The model under review builds one solid part; all positions refer to its coordinate system, in mm. Face numbers are marked on the shaded views. A direction names the side the tool comes from. Round coordinates to 2 decimals unless told otherwise and drop trailing zeros. Write each loop counter-clockwise with the first axis right and the second up, starting at its lowest first coordinate (ties: lowest second). Pieces come first, ordered by that corner, then holes.
Item 1: Add section C-C (x = -16). Give the boundary of the cut face in (y, z), plus the area to 3 significant figures.
Item 2: Add section A-A (z = 13). Give the boundary of the cut face in (x, y), plus the area to 3 significant figures.
Item 3: Add section B-B (y = 8.75). Give the boundary of the cut face in (x, z).
Item 4: Add section D-D (z = 33). Give the boundary of the cut face in (x, y).
Item 5: Machinability: for the marked faces 1, 2 and 3, which of the approach directions +Z, -Z, +X, -X, +Y, -Y give a long, thin tool a straight path to every point of the face, cutting with its end or side? Answer none if there is none.
Item 6: Clearance check with flat-ended pins moving along their axes: pin 1 Ø11.5 at (x, z) = (-57.5, 15.5) entering from -Y; pin 2 Ø5 at (y, z) = (1.5, 42.5) entering from -X; pin 3 Ø9 at (x, y) = (-95, 9) entering from +Z; pin 4 Ø5 at (y, z) = (1.5, 22) entering from -X. State where each tip first meets the part, or that it passes through.
Item 7: To check wall thickness, follow L1, parallel to X at y = 14.5, z = 41; L2, parallel to Z at x = -39, y = 7.5; L3, parallel to X at y = 9, z = 25. State the ranges of each line that lie inside material, in increasing order.
```python
from build123d import *

# Parameters (mm, degrees)
EXTRUDE_1_DEPTH     = 60
SKETCH_2_W          = 5
SKETCH_2_H          = 8
EXTRUDE_2_DEPTH     = 175
CHAMFER_1_SIZE      = 20
CUT_EXTRUDE_1_DEPTH = 33.8
CHAMFER_2_SIZE      = 2


with BuildPart() as part:
    # 草图1 → 凸台-拉伸1 (new body)
    with BuildSketch(Plane.XY):
        Polygon((5.6, 10.6), (3.2, 10.6), (3.2, 15.2), (0, 15.2), (0, 0), (3.2, 0), (3.2, 4.6), (5.6, 4.6), (5.6, -2.4), (-2.4, -2.4), (-2.4, 17.6), (5.6, 17.6), align=None)
    extrude(amount=EXTRUDE_1_DEPTH)

    # 草图2 → 凸台-拉伸2 (add)
    with BuildSketch(Plane.ZY.offset(2.4)):
        with Locations((2.5, 7.6)):
            Rectangle(SKETCH_2_W, SKETCH_2_H)
    extrude(amount=EXTRUDE_2_DEPTH)

    # 倒角1
    chamfer_1_edges = [part.edges().sort_by_distance(p)[0] for p in [
        (-2.4, 7.6, 5),
    ]]
    chamfer(chamfer_1_edges, length=CHAMFER_1_SIZE)

    # 草图3 → 切除-拉伸1 (cut)
    with BuildSketch(Plane(origin=(0, 11.6, 0), x_dir=(1, 0, 0), z_dir=(0, 1, 0))):
        Polygon((-177.4, -2.5), (-157.4, -5), (-177.4, -5), align=None)
    extrude(amount=-CUT_EXTRUDE_1_DEPTH, mode=Mode.SUBTRACT)

    # 倒角2
    chamfer_2_edges = [part.edges().sort_by_distance(p)[0] for p in [
        (-2.4, 3.6, 12.5),
        (-2.4, 11.6, 12.5),
    ]]
    chamfer(chamfer_2_edges, length=CHAMFER_2_SIZE)


solid = part.part
```
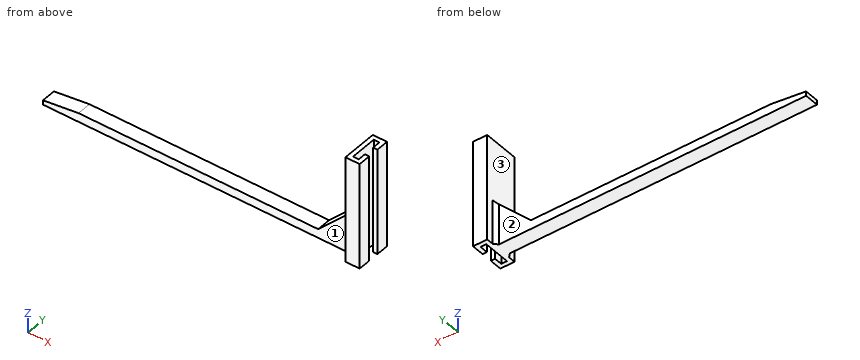
Numbers:
1. outline: (3.6, 0) - (11.6, 0) - (11.6, 11.4) - (3.6, 11.4) - close
1. area: 91.2 mm2
2. outline: (-14.4, 3.6) - (-4.4, 3.6) - (-2.4, 1.6) - (-2.4, -2.4) - (5.6, -2.4) - (5.6, 4.6) - (3.2, 4.6) - (3.2, 0) - (0, 0) - (0, 15.2) - (3.2, 15.2) - (3.2, 10.6) - (5.6, 10.6) - (5.6, 17.6) - (-2.4, 17.6) - (-2.4, 13.6) - (-4.4, 11.6) - (-14.4, 11.6) - close
2. area: 197 mm2
3. outline: (-177.4, 0) - (0, 0) - (0, 60) - (-2.4, 60) - (-2.4, 25) - (-22.4, 5) - (-157.4, 5) - (-177.4, 2.5) - close
4. outline: (-2.4, -2.4) - (5.6, -2.4) - (5.6, 4.6) - (3.2, 4.6) - (3.2, 0) - (0, 0) - (0, 15.2) - (3.2, 15.2) - (3.2, 10.6) - (5.6, 10.6) - (5.6, 17.6) - (-2.4, 17.6) - close
5. face 1: +Z, -Z, -X, -Y
5. face 2: +Z, -Z, -X, +Y
5. face 3: +Z, -X
6. pin 1: passes through
6. pin 2: stops at x = -2.4
6. pin 3: stops at z = 5
6. pin 4: stops at x = -6.76
7. L1: x = -2.4 to 0, 3.2 to 5.6
7. L2: z = 0 to 5
7. L3: x = -2.4 to 0
